The figure shows three views and two pictorial views of one solid part (mm, origin at its lowest corner). Answer the questions. Round coordinates to 2 decimals unless told otherwise and drop trailing zeros. Order: outer loops, then holes, each group sorted by start corner. A loop starts at its lowest first (then second) coordinate and runs counter-clockwise, first axis right, second up. Notation, with made-up numbers: (7.5, 60.25) - (36.5, 60.25) arc R13 ccw to (36.5, 66.25) - close; hole circle Ø2 at (75, -12.75). An arc over 180 degrees is marked (long way). One line per item, written item: value. Start each with the question number.
1. A flat-ended cylindrical pin translates along its axis: P1, Ø3.5, axis at x = 15, y = 29, coming from the +Z side. Find the tip coordinate at first contact, or state that the pin passes through.
2. Section B-B, the plane y = 49 is taken. Give the vertices of the cut face in (x, z).
3. Section C-C, the plane x = 15 is taken. Give the vertices of the cut face in (y, z), then the cut area to 3 significant figures.
4. Straight lines are drawn through the part: line 1 (Y direction, x = 110, z = 6.25); line 2 (Y direction, x = 180, z = 6); line 3 (Y direction, x = 150, z = 3.75). For each, find the intervals that lie inside material, in ascending order.
5. Section A-A, the plane x = 110 is taken. Give the vertices of the cut face in (y, z).
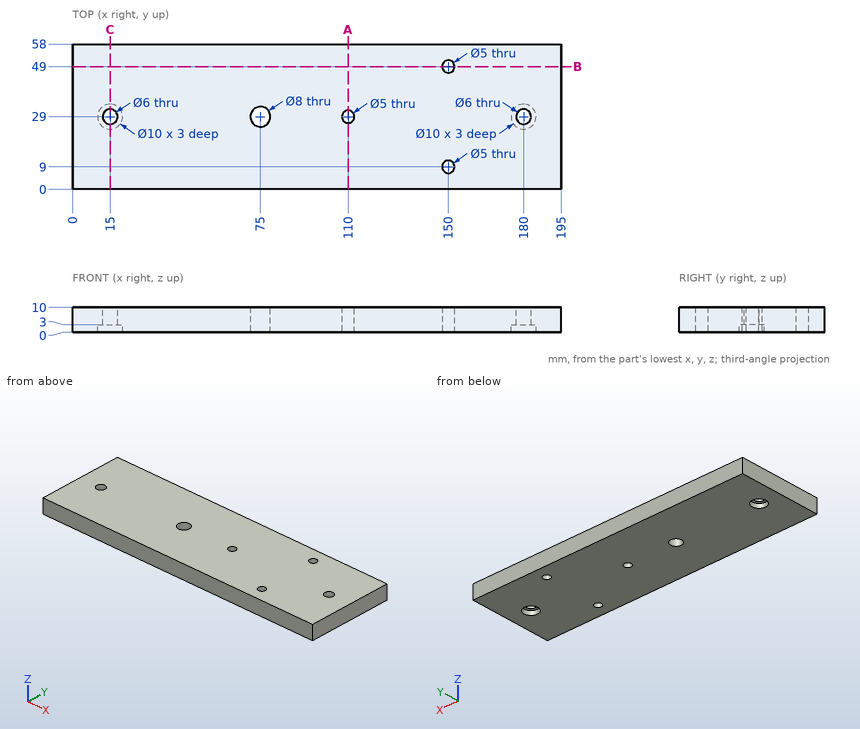
Answer list:
1. P1: passes through
2. outline: (0, 0) - (147.5, 0) - (147.5, 10) - (0, 10) - close; (152.5, 0) - (195, 0) - (195, 10) - (152.5, 10) - close
3. outline: (0, 0) - (24, 0) - (24, 3) - (26, 3) - (26, 10) - (0, 10) - close; (32, 3) - (34, 3) - (34, 0) - (58, 0) - (58, 10) - (32, 10) - close
3. area: 508 mm²
4. line 1: y = 0 to 26.5, 31.5 to 58
4. line 2: y = 0 to 26, 32 to 58
4. line 3: y = 0 to 6.5, 11.5 to 46.5, 51.5 to 58
5. outline: (0, 0) - (26.5, 0) - (26.5, 10) - (0, 10) - close; (31.5, 0) - (58, 0) - (58, 10) - (31.5, 10) - close
